from build123d import *

# Parameters (mm, degrees)
CUT_EXTRUDE1_DEPTH      = 40.347808071
CUT_EXTRUDE1_DEPTH_BACK = 40.347808071
SKETCH2_R               = 3.5
SKETCH3_R               = 7.5
CUT_EXTRUDE2_DEPTH      = 5


with BuildPart() as part:
    # Sketch1 → Revolve1 (revolve)
    with BuildSketch(Plane.XY, mode=Mode.PRIVATE) as revolve1_sk:
        Polygon((-9.5, 0), (9.5, 0), (9.5, 27), (7.5, 27), (7.5, 25), (-2.5, 25), (-2.5, 27), (-4.5, 27), (-4.5, 5), (-9.5, 5), align=None)
    revolve(revolve1_sk.sketch.rotate(Axis((-9.5, 0, 0), (1, 0, 0)), 90), axis=Axis((-9.5, 0, 0), (1, 0, 0)))

    # Sketch2 → Cut-Extrude1 (cut, two sides: drawn at the far end of the back side and taken through both)
    with BuildSketch(Plane(origin=(0, 0, 0), x_dir=(0, 0, -1), z_dir=(1, 0, 0)).offset(-CUT_EXTRUDE1_DEPTH_BACK)):
        Circle(SKETCH2_R)
    extrude(amount=CUT_EXTRUDE1_DEPTH + CUT_EXTRUDE1_DEPTH_BACK, mode=Mode.SUBTRACT)

    # Sketch3 → Cut-Extrude2 (cut)
    with BuildSketch(Plane(origin=(9.5, 0, 0), x_dir=(0, 0, -1), z_dir=(1, 0, 0))):
        Circle(SKETCH3_R)
    extrude(amount=-CUT_EXTRUDE2_DEPTH, mode=Mode.SUBTRACT)


solid = part.part
Work out the finished part from the listing and answer in its coordinate system (mm). A direction names the side the tool comes from. Give positions to 0.01 mm unless a question says otherwise; leave off trailing zeros. Loops run counter-clockwise (first coordinate to the right, second up) from the corner with the lowest first, then second, coordinate; pieces in that order, holes last. Notation, with made-up numbers: (-39.75, -10.5) - (-10.75, -10.5) arc R29 ccw to (-10.75, 9.5) - close; hole circle Ø11 at (45, -32.5). An arc over 180 degrees is marked (long way). Answer in a Markdown table with one row per item. Add a question column.
Q1. A tool of negligible diameter and unlimited length cuts with its end or side. For faces 1 (the cylindrical face through (7.035, 0.33, 7.493)), 2 (the cylindrical face through (-7, 0, -5)), 3 (the cylindrical face through (2.43, -7.509, 23.846)), from which of +Z, -Z, +X, -X, +Y, -Y can it reach the whole face along a straight path? Write none if from no direction.
Q2. The part is cut by section C-C (x = 0). Determine the outline of the cut face in (y, z).
Q3. The part is cut by section D-D (y = -12). Determine the outline of the cut face in (x, z).
Q4. Determine the mould class of faces 4 (the flat face through (7.5, 8, 24)), 5 (the flat face through (-9.5, 3.3, 2.2)), 6 (the cylindrical face through (-2.598, -1.341, -3.233)) for opening direction X: released by +X, released by -X, zero draft, split by the parting line, or undercut.
Q5. Consider line 1 along Y through (x, z) = (-0.25, 0); line 2 along Y through (x, z) = (7.05, 0); line 3 along X through (y, z) = (1, -6). Determine where each line is inside the solid, lowest interval first.
Q6. The part is cut by section A-A (y = 0). Determine the outline of the cut face in (x, z), and give its area (3 significant figures).
Q7. Each of these flat-tipped pins is pushed along its axis until it touches: P1, Ø4, axis at x = -2, y = -12.5, coming from the -Z side; P2, Ø4, axis at x = 1, z = -9, coming from the +Y side; P3, Ø10, axis at y = -19.5, z = -9, coming from the -X side. Where does it stop, or does it pass through?
Solution:
| question | item | result |
|---|---|---|
| 1 | face 1 | +X |
| 1 | face 2 | -X |
| 1 | face 3 | none |
| 2 | outline | circle Ø50 at (0, 0); hole circle Ø7 at (0, 0) |
| 3 | outline | (-4.5, -24.19) - (-2.5, -24.19) - (-2.5, -21.93) - (7.5, -21.93) - (7.5, -24.19) - (9.5, -24.19) - (9.5, 24.19) - (7.5, 24.19) - (7.5, 21.93) - (-2.5, 21.93) - (-2.5, 24.19) - (-4.5, 24.19) - close |
| 4 | face 4 | undercut |
| 4 | face 5 | released by -X |
| 4 | face 6 | zero draft |
| 5 | line 1 | y = -25 to -3.5, 3.5 to 25 |
| 5 | line 2 | y = -25 to -7.5, 7.5 to 25 |
| 5 | line 3 | x = -4.5 to 4.5 |
| 6 | outline | (-9.5, -5) - (-4.5, -5) - (-4.5, -27) - (-2.5, -27) - (-2.5, -25) - (7.5, -25) - (7.5, -27) - (9.5, -27) - (9.5, -7.5) - (4.5, -7.5) - (4.5, -3.5) - (-9.5, -3.5) - close; (-9.5, 3.5) - (4.5, 3.5) - (4.5, 7.5) - (9.5, 7.5) - (9.5, 27) - (7.5, 27) - (7.5, 25) - (-2.5, 25) - (-2.5, 27) - (-4.5, 27) - (-4.5, 5) - (-9.5, 5) - close |
| 6 | area | 593 mm² |
| 7 | P1 | stops at z = -24.85 |
| 7 | P2 | stops at y = 24 |
| 7 | P3 | stops at x = -4.5 |
